Source: CAD feature listing. Evaluate the final solid. Frame: model axes, mm. A direction names the side the tool comes from. Coordinates: 2 decimals unless noted, no trailing zeros. Order: outer loops, then holes, each group sorted by start corner. A loop starts at its lowest first (then second) coordinate and runs counter-clockwise, first axis right, second up.
Item 1: Mould query, pull axis X, two halves, no side actions, for faces 5 (the cylindrical face through (21.803, -2.814, -1.03)), 6 (the cylindrical face through (-21.864, -2.753, -1.03)), 7 (the cylindrical face through (18.035, 0.067, -1.03)), 8 (the cylindrical face through (-21.08, 0.07, -1.03)). Classes: released by +X, released by -X, zero draft, split by the parting line, or undercut.
Item 2: Contact query for flat-ended pins moving along their axis: P1, Ø16, axis at x = 5.5, y = -7, coming from the +Z side; P2, Ø6, axis at x = 19, y = 1.5, coming from the -Z side; P3, Ø1, axis at y = 1.5, z = -19.5, coming from the +X side. Output: stop coordinate, or through.
Item 3: Section B-B on z = -1.5. State how many separate pieces and enclosed holes the cut face has, then the cut area to 3 significant figures.
Item 4: Section C-C on x = 20. Return the cut outline in (y, z), then the cut area to 3 significant figures.
Item 5: Reachability of faces 1 (the flat face through (-17, -3.937, -1)), 2 (the flat face through (-17, 3.937, -1)), 3 (the flat face through (17, 3.937, -1)), 4 (the flat face through (-6, -12, -11.43)) from +Z, -Z, +X, -X, +Y, -Y: full face, straight path, thin tool, end or side. Return the list, or none.
Item 6: Section D-D on y = -4.5. Return the cut outline in (x, z).
Item 7: Ray query, line 1 (X direction, y = 0, z = -1); line 2 (Y direction, x = 0, z = 6.75) (3 decimals); line 3 (Z direction, x = -10.5, y = 3.5). Return the intervals inside material, ascending.
from build123d import *

# Parameters (mm, degrees)
SKETCH1_R               = 16.002
BOSS_EXTRUDE1_DEPTH     = 13.97
SKETCH2_R               = 11.938
BOSS_EXTRUDE2_DEPTH     = 9.906
CUT_EXTRUDE1_START      = -2.54
SKETCH3_R               = 16.002
SKETCH3_R_2             = 13.208
CUT_EXTRUDE1_DEPTH      = 2.54
SKETCH4_W               = 45.974
SKETCH4_H               = 7.874
BOSS_EXTRUDE3_DEPTH     = 2.032
CUT_EXTRUDE2_DEPTH      = 37.803933879
CUT_EXTRUDE2_DEPTH_BACK = 37.803933879
SKETCH5_R               = 1.524
FILLET1_R               = 3.937
SKETCH6_R               = 4.572
BOSS_EXTRUDE4_DEPTH     = 0.508
SKETCH7_R               = 3.937
BOSS_EXTRUDE5_DEPTH     = 2.032
SKETCH8_R               = 2.413
BOSS_EXTRUDE6_DEPTH     = 9.906
CUT_EXTRUDE3_DEPTH      = 44.88268106
CUT_EXTRUDE3_DEPTH_BACK = 5.08
SKETCH10_R              = 1.143
CUT_EXTRUDE4_DEPTH      = 7.874


with BuildPart() as part:
    # Sketch1 → Boss-Extrude1 (new body)
    with BuildSketch(Plane.XY):
        Circle(SKETCH1_R)
    extrude(amount=-BOSS_EXTRUDE1_DEPTH)

    # Sketch2 → Boss-Extrude2 (add)
    with BuildSketch(Plane(origin=(0, 0, -13.97), x_dir=(-1, 0, 0), z_dir=(0, 0, -1))):
        Circle(SKETCH2_R)
    extrude(amount=BOSS_EXTRUDE2_DEPTH)

    # Sketch3 → Cut-Extrude1 (cut)
    with BuildSketch(Plane(origin=(0, 0, -13.97), x_dir=(-1, 0, 0), z_dir=(0, 0, -1)).offset(CUT_EXTRUDE1_START)):
        with Locations(Location((0, 0, 0), (0, 0, 180))):
            Circle(SKETCH3_R)
        Circle(SKETCH3_R_2, mode=Mode.SUBTRACT)
    extrude(amount=CUT_EXTRUDE1_DEPTH, mode=Mode.SUBTRACT)

    # Sketch4 → Boss-Extrude3 (add)
    with BuildSketch(Plane.XY):
        Rectangle(SKETCH4_W, SKETCH4_H)
    extrude(amount=-BOSS_EXTRUDE3_DEPTH)

    # Sketch5 → Cut-Extrude2 (cut, two sides: drawn at the far end of the back side and taken through both)
    with BuildSketch(Plane.XY.offset(-CUT_EXTRUDE2_DEPTH_BACK)):
        with Locations((-19.558, 0)):
            Circle(SKETCH5_R)
        with Locations((19.558, 0)):
            Circle(SKETCH5_R)
    extrude(amount=CUT_EXTRUDE2_DEPTH + CUT_EXTRUDE2_DEPTH_BACK, mode=Mode.SUBTRACT)

    # Fillet1
    fillet1_edges = [part.edges().sort_by_distance(p)[0] for p in [
        (22.987, 3.937, -1.016),
        (22.987, -3.937, -1.016),
        (-22.987, -3.937, -1.016),
        (-22.987, 3.937, -1.016),
    ]]
    fillet(fillet1_edges, radius=FILLET1_R - 0.0001)  # a hair under: the kernel refuses the full size

    # Sketch6 → Boss-Extrude4 (add)
    with BuildSketch(Plane.XY):
        with Locations((0, 9.398)):
            Circle(SKETCH6_R)
    extrude(amount=BOSS_EXTRUDE4_DEPTH)

    # Sketch7 → Boss-Extrude5 (add)
    with BuildSketch(Plane.XY):
        with Locations((0, 9.398)):
            Circle(SKETCH7_R)
    extrude(amount=BOSS_EXTRUDE5_DEPTH)

    # Sketch8 → Boss-Extrude6 (add)
    with BuildSketch(Plane.XY):
        with Locations((0, 9.398)):
            Circle(SKETCH8_R)
    extrude(amount=BOSS_EXTRUDE6_DEPTH)

    # Sketch9 → Cut-Extrude3 (cut, two sides: drawn at the far end of the back side and taken through both)
    with BuildSketch(Plane.XY.offset(9.906).offset(-CUT_EXTRUDE3_DEPTH_BACK)):
        with BuildLine():
            Line((-1.481061781, 11.303), (1.481061781, 11.303))
            ThreePointArc((1.481061781, 11.303), (0, 11.811), (-1.481061781, 11.303))
        make_face()
        with BuildLine():
            Line((-1.481061781, 7.493), (1.481061781, 7.493))
            ThreePointArc((1.481061781, 7.493), (0, 6.985), (-1.481061781, 7.493))
        make_face()
    extrude(amount=CUT_EXTRUDE3_DEPTH + CUT_EXTRUDE3_DEPTH_BACK, mode=Mode.SUBTRACT)

    # Sketch10 → Cut-Extrude4 (cut)
    with BuildSketch(Plane.XY.offset(9.906)):
        with Locations((0, 9.398)):
            Circle(SKETCH10_R)
    extrude(amount=-CUT_EXTRUDE4_DEPTH, mode=Mode.SUBTRACT)


solid = part.part
Answer list:
1. face 5: released by +X
1. face 6: released by -X
1. face 7: undercut
1. face 8: undercut
2. P1: stops at z = 0
2. P2: stops at z = -2.03
2. P3: stops at x = 11.9
3. separate pieces: 1
3. enclosed holes: 2
3. area: 889 mm2
4. outline: (-3.82, -2.03) - (-1.46, -2.03) - (-1.46, 0) - (-3.82, 0) - close; (1.46, -2.03) - (3.82, -2.03) - (3.82, 0) - (1.46, 0) - close
4. area: 9.60 mm2
5. face 1: +Z, -Z, -X, -Y
5. face 2: +Z, -Z, -X, +Y
5. face 3: +Z, -Z, +X, +Y
5. face 4: -Z
6. outline: (-15.36, -11.43) - (-12.42, -11.43) - (-12.42, -13.97) - (-11.06, -13.97) - (-11.06, -23.88) - (11.06, -23.88) - (11.06, -13.97) - (12.42, -13.97) - (12.42, -11.43) - (15.36, -11.43) - (15.36, 0) - (-15.36, 0) - close
7. line 1: x = -22.99 to -21.08, -18.03 to 18.03, 21.08 to 22.99
7. line 2: y = 7.493 to 8.255, 10.541 to 11.303
7. line 3: z = -23.88 to 0
